The figure shows three views and two pictorial views of one solid part (mm, origin at its lowest corner). Answer the questions. Coordinates: 2 decimals unless noted, no trailing zeros. Write each loop counter-clockwise with the first axis right and the second up, starting at its lowest first coordinate (ties: lowest second). Pieces come first, ordered by that corner, then holes. Notation, with made-up numbers: M 23.25,13.5 L 72.25,13.5 A6 cw 72.25,19.5 Z; hole C 40.25,-27.75 d9. An arc over 180 degrees is marked long. Write item = value, one per line.
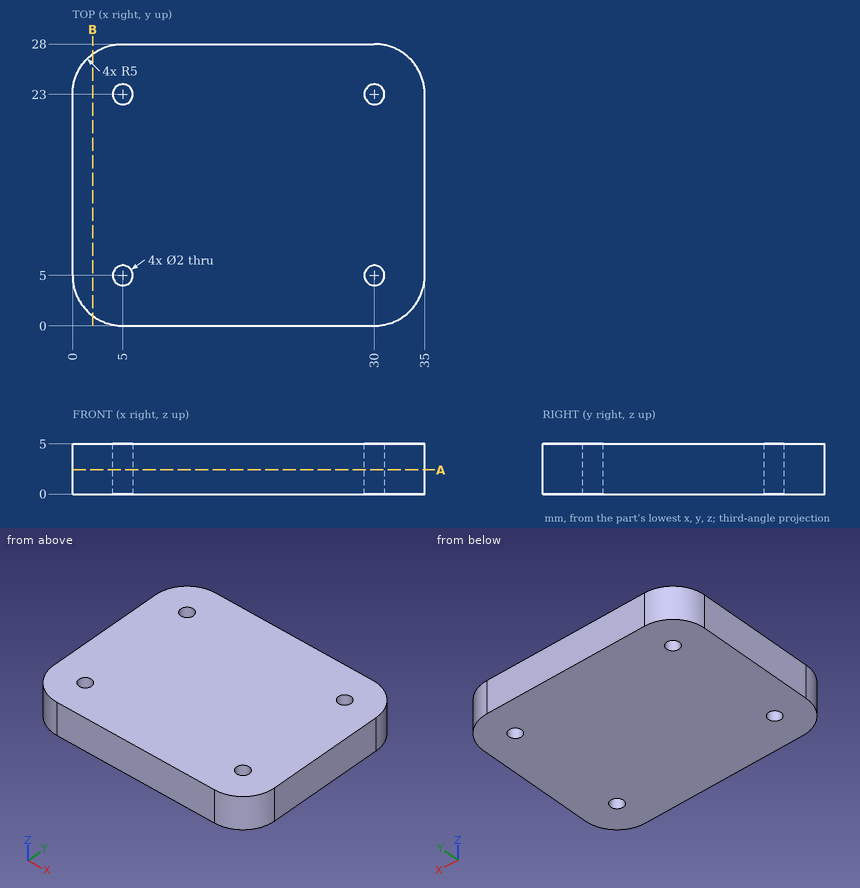
Item 1: Flat-ended cylindrical pins translate along their axes: pin 1 (1.8 mm diameter, centred on x = 5, y = 23, fed in from -Z); pin 2 (2.5 mm diameter, centred on x = 5, y = 5, fed in from -Z). Find the tip coordinate at first contact, or state that the pin passes through.
Worked answers:
pin_1 = through
pin_2 = 0
Item 2: Find section A-A (z = 2.4). Determine the outline of the cut face in (x, y).
Worked answers:
outline = M 0,5 A5 ccw 5,0 L 30,0 A5 ccw 35,5 L 35,23 A5 ccw 30,28 L 5,28 A5 ccw 0,23 Z; hole C 5,5 d2; hole C 5,23 d2; hole C 30,5 d2; hole C 30,23 d2
Item 3: Consider line 1 along Y through (x, z) = (30, 1.45); line 2 along X through (y, z) = (1.75, 4.55); line 3 along Y through (x, z) = (3, 0.6). Determine where each line is inside the solid, lowest interval first. Write a range as from..to.
Worked answers:
line_1 = 0..4, 6..22, 24..28
line_2 = 1.2..33.8
line_3 = 0.42..27.58
Item 4: Find section B-B (x = 2). Determine the outline of the cut face in (y, z), and give its area (3 significant figures).
Worked answers:
outline = M 1,0 L 27,0 L 27,5 L 1,5 Z
area = 130 mm²
